The listing builds one solid part. Answer for the finished solid, in the listing's coordinates (mm). Face numbers are marked on the shaded views. Round coordinates to 2 decimals unless told otherwise and drop trailing zeros. Loops run counter-clockwise (first coordinate to the right, second up) from the corner with the lowest first, then second, coordinate; pieces in that order, holes last. Notation, with made-up numbers: (-35, 32.5) -> (-27, 32.5) arc R32 cw to (-27, 71.5) -> close; hole circle Ø9 at (37.5, 77). An arc over 180 degrees is marked (long way). Write each question's results on one line, items separated by ' | '. Start each with the question number.
(1) The part is cut by section A-A (y = 0). Determine the outline of the cut face in (x, z), plus the area to 3 significant figures.
(2) Determine the mould class of the marked faces 1, 2, 3 and 4 for opening direction X: released by +X, released by -X, zero draft, split by the parting line, or undercut.
(3) The part is cut by section B-B (x = 27.5). Determine the outline of the cut face in (y, z), plus the area to 4 significant figures.
(4) The part is cut by section C-C (x = 0). Count the separate pieces of the cut face and the enclosed holes in it, plus the area to 3 significant figures.
(5) Straight lines are drawn through the part: probe 1 along Y at (x, z) = (0, -1.2); probe 2 along X at (y, z) = (23, 1); probe 3 along Y at (x, z) = (-19, 1). For each, find the intervals that lie inside material, in ascending order.
(6) Flat-ended cylindrical pins translate along their axes: pin 1 (5 mm diameter, centred on x = -18.5, y = 16.5, fed in from +Z); pin 2 (1 mm diameter, centred on y = 30, z = 3.5, fed in from +X); pin 3 (1.6 mm diameter, centred on x = -39.5, z = 4.5, fed in from +Y); pin 4 (5 mm diameter, centred on x = 0, y = 0, fed in from -Z). Find the tip coordinate at first contact, or state that the pin passes through.
(7) The part is cut by section D-D (y = 14). Determine the outline of the cut face in (x, z).
```python
from build123d import *

# Parameters (mm, degrees)
F0_W                   = 85
F0_H                   = 65
F0_W_2                 = 77
F0_H_2                 = 57
F1_DEPTH               = 5
F2_DEPTH               = 5
F3_W                   = 10
F3_H                   = 4
F3_W_2                 = 40
F3_W_3                 = 4
F3_H_2                 = 20.5
F4_DEPTH               = 4
F5_T1_DEPTH            = 4
F5_T3_DEPTH            = 4
F6_R                   = 2
F8_D                   = 6.8
F8_CBORE_D             = 7.5
F8_CBORE_DEPTH         = 1.5
F9_R                   = 9
F9_R_2                 = 3.25
F10_DEPTH              = 3
F11_DEPTH              = 25
F12_R                  = 5
F15_D                  = 3
F15_CBORE_D            = 6
F15_CBORE_DEPTH        = 3
F15_ON_F13_D           = 3
F15_ON_F13_CBORE_D     = 6
F15_ON_F13_CBORE_DEPTH = 3


# Not quite as in the source:
# - a fillet or chamfer that OpenCascade refuses, or shapes differently, is made with other operations: its cross-section is extruded or revolved along the edge and cut away or added


with BuildPart() as f1:
    # F0 (on Top) → F1 (new body)
    with BuildSketch(Plane.XY):
        Rectangle(F0_W, F0_H)
        Rectangle(F0_W_2, F0_H_2, mode=Mode.SUBTRACT)
        Rectangle(F0_W_2, F0_H_2)
    extrude(amount=-F1_DEPTH)

    # F0 (on Top) → F2 (join)
    with BuildSketch(Plane.XY):
        Rectangle(F0_W, F0_H)
        Rectangle(F0_W_2, F0_H_2, mode=Mode.SUBTRACT)
    extrude(amount=F2_DEPTH)

    # F3 (on face) → F4 (cut)
    with BuildSketch(Plane.XY.offset(5)):
        with Locations((28.5, 30.5)):
            Rectangle(F3_W, F3_H)
        with Locations((0, 30.5)):
            Rectangle(F3_W_2, F3_H)
        with Locations((0, -30.5)):
            Rectangle(F3_W_2, F3_H)
        with Locations((-28.5, -30.5)):
            Rectangle(F3_W, F3_H)
        with Locations((-40.5, 14.25)):
            Rectangle(F3_W_3, F3_H_2)
        with Locations((40.5, -14.25)):
            Rectangle(F3_W_3, F3_H_2)
    extrude(amount=-F4_DEPTH, mode=Mode.SUBTRACT)

    # F5: fillet of radius 15 on 4 edges, made by hand

    # F5_s2 → F5_t1 (join)
    with BuildSketch(Plane.XZ.offset(-32.5)):
        with BuildLine():
            ThreePointArc((-9.8019609728, 1), (-15.2791865479, 2.0357599562), (-20, 5))
            Line((-20, 5), (-20, 1))
            Line((-20, 1), (-9.8019609728, 1))
        make_face()
        with BuildLine():
            ThreePointArc((20, 5), (15.2791865479, 2.0357599562), (9.8019609728, 1))
            Line((9.8019609728, 1), (20, 1))
            Line((20, 1), (20, 5))
        make_face()
    extrude(amount=F5_T1_DEPTH)

    # F5_s4 → F5_t3 (join)
    with BuildSketch(Plane.XZ.offset(28.5)):
        with BuildLine():
            ThreePointArc((9.8019609728, 1), (15.2791865479, 2.0357599562), (20, 5))
            Line((20, 5), (20, 1))
            Line((20, 1), (9.8019609728, 1))
        make_face()
        with BuildLine():
            ThreePointArc((-20, 5), (-15.2791865479, 2.0357599562), (-9.8019609728, 1))
            Line((-9.8019609728, 1), (-20, 1))
            Line((-20, 1), (-20, 5))
        make_face()
    extrude(amount=F5_T3_DEPTH)

    # F6
    f6_edges = [f1.edges().sort_by_distance(p)[0] for p in [
        (40.5, -4, 1),
        (40.5, -24.5, 1),
        (-40.5, 24.5, 1),
        (-40.5, 4, 1),
        (-33.5, -30.5, 1),
        (-23.5, -30.5, 1),
        (33.5, 30.5, 1),
        (23.5, 30.5, 1),
    ]]
    fillet(f6_edges, radius=F6_R)

    # F8 (through all)
    with Locations(Plane.XY):
        with Locations((0, 24), (0, -24)):
            CounterBoreHole(F8_D / 2, F8_CBORE_D / 2, F8_CBORE_DEPTH)

    # F9 (on face) → F10 (cut)
    with BuildSketch(Plane.XY):
        Circle(F9_R)
        Circle(F9_R_2, mode=Mode.SUBTRACT)
    extrude(amount=-F10_DEPTH, mode=Mode.SUBTRACT)

    # F9 (on face) → F11 (cut)
    with BuildSketch(Plane.XY):
        Circle(F9_R_2)
    extrude(amount=-F11_DEPTH, mode=Mode.SUBTRACT)

    # F12
    f12_edges = [f1.edges().sort_by_distance(p)[0] for p in [
        (42.5, -32.5, 0),
        (42.5, 32.5, 0),
        (-42.5, -32.5, 0),
        (-42.5, 32.5, 0),
    ]]
    fillet(f12_edges, radius=F12_R)

    # F15 (through all)
    with Locations(Plane(origin=(0, 32.5, 0), x_dir=(-1, 0, 0), z_dir=(0, 1, 0))):
        with Locations((27.5, 2.5)):
            CounterBoreHole(F15_D / 2, F15_CBORE_D / 2, F15_CBORE_DEPTH)

    # F15 on F13 (through all)
    with Locations(Plane.XZ.offset(32.5)):
        with Locations((27.5, 2.5)):
            CounterBoreHole(F15_ON_F13_D / 2, F15_ON_F13_CBORE_D / 2, F15_ON_F13_CBORE_DEPTH)


solid = f1.part
```
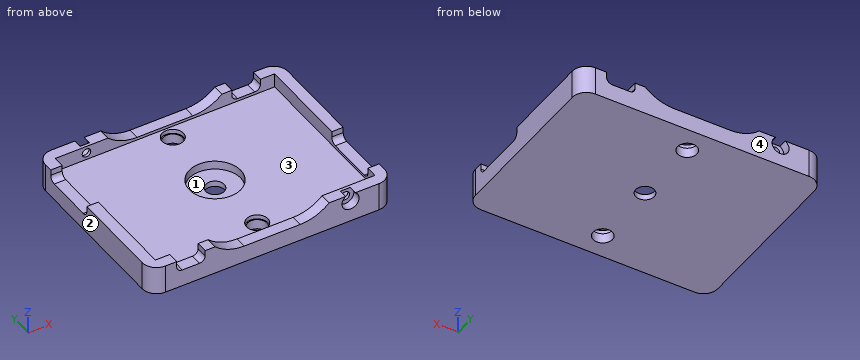
Checked values:
1) outline: (-42.5, -5) -> (-3.25, -5) -> (-3.25, -3) -> (-9, -3) -> (-9, 0) -> (-38.5, 0) -> (-38.5, 5) -> (-42.5, 5) -> close; (3.25, -5) -> (42.5, -5) -> (42.5, 5) -> (38.5, 5) -> (38.5, 0) -> (9, 0) -> (9, -3) -> (3.25, -3) -> close | area: 398 mm2
2) face 1: undercut | face 2: released by -X | face 3: undercut | face 4: zero draft
3) outline: (-32.5, -5) -> (32.5, -5) -> (32.5, 1) -> (28.5, 1) -> (28.5, 0) -> (-28.5, 0) -> (-28.5, 1) -> (-29.5, 1) -> (-29.5, -0.5) -> (-32.5, -0.5) -> close; (-29.5, 4) -> (-28.5, 4) -> (-28.5, 5) -> (-29.5, 5) -> close | area: 329.5 mm2
4) separate pieces: 4 | enclosed holes: 0 | area: 196 mm2
5) probe 1: y = -32.5 to -27.75, -20.25 to -9, 9 to 20.25, 27.75 to 32.5 | probe 2: x = -42.5 to -38.5, 38.5 to 42.5 | probe 3: y = -32.5 to -28.5, 28.5 to 32.5
6) pin 1: stops at z = 0 | pin 2: stops at x = 42.08 | pin 3: stops at y = 32.35 | pin 4: passes through
7) outline: (-42.5, -5) -> (42.5, -5) -> (42.5, 5) -> (38.5, 5) -> (38.5, 0) -> (-38.5, 0) -> (-38.5, 1) -> (-42.5, 1) -> close
